Study the drawing (mm; zero at the part's minimum x, y, z) and answer. Give positions to 0.01 mm unless a question says otherwise; leave off trailing zeros. Loops run counter-clockwise (first coordinate to the right, second up) from the corner with the lowest first, then second, coordinate; pieces in that order, holes last. Notation, with made-up numbers: M 20,-32 L 62,-32 A9 cw 62,-28 Z; hole C 37,79.25 d6. An arc over 180 degrees is marked long. Return JSON: item names as keys, results as strings.
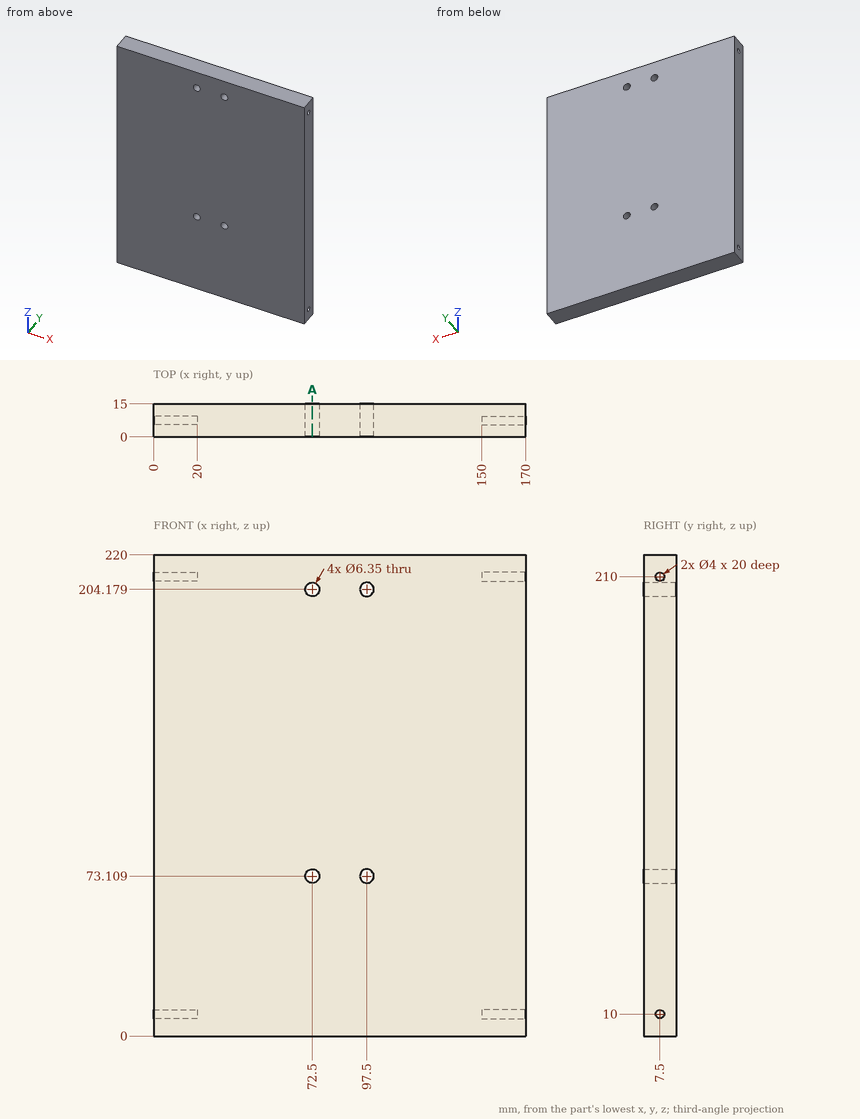
(1) Straight lines are drawn through the part: line 1 along Y through (x, z) = (9, 10); line 2 along Z through (x, y) = (71, 6). For each, find the intervals that lie inside material, in ascending order.
Values follow:
{"line 1": "0 to 5.5, 9.5 to 15", "line 2": "0 to 70.31, 75.91 to 201.38, 206.98 to 220"}
(2) The part is cut by section A-A (x = 72.5). Determine the outline of the cut face in (y, z), and give its area (3 significant figures).
Values follow:
{"outline": "M 0,0 L 15,0 L 15,69.93 L 0,69.93 Z; M 0,76.28 L 15,76.28 L 15,201 L 0,201 Z; M 0,207.35 L 15,207.35 L 15,220 L 0,220 Z", "area": "3,110 mm²"}
(3) Given pin 1 (3.5 mm diameter, centred on y = 7.5, z = 10, fed in from -X); pin 2 (5 mm diameter, centred on y = 7.5, z = 210, fed in from -X); pin 3 (3 mm diameter, centred on y = 7.5, z = 10, fed in from +X), each flat-ended and moving along its own axis, determine where each tip first touches the part or whether it passes through.
Values follow:
{"pin 1": "x = 20", "pin 2": "x = 0", "pin 3": "x = 150"}
